Autodesk Inventor part; units mm, degrees
ref_plane "YZ Plane" through (0, 0, 0) normal (1, 0, 0) x (0, 1, 0)
ref_plane "XZ Plane" through (0, 0, 0) normal (0, 1, 0) x (-1, 0, 0)
ref_plane "XY Plane" through (0, 0, 0) normal (0, 0, 1) x (1, 0, 0)
sketch "Sketch1" plane through (0, 0, 0) normal (0, 0, 1) x (1, 0, 0)
  line L0 (0, 0) -> (175, 0)
  line L1 (0, 0) -> (0, 68)
  line L2 (0, 68) -> (-5, 68)
  line L3 (-5, 68) -> (-5, -5)
  line L4 (-5, -5) -> (180, -5)
  line L5 (180, -5) -> (180, 68)
  line L6 (180, 68) -> (175, 68)
  line L7 (175, 68) -> (175, 0)
  dimension "d0" = 175
  dimension "d1" = 68
  dimension "d2" = 5
  dimension "d3" = 73
  dimension "d4" = 185
  dimension "d5" = 73
  dimension "d6" = 5
extrude "Outline" add sketch "Sketch1" along normal blind 30
sketch "Sketch2" plane through (-5, -5, 0) normal (-1, 0, 0) x (0, 0, 1)
  line L0 (0, 73) -> (30, 73) construction
  line L1 (15, 73) -> (15, 43) construction
  line L2 (5, 22.5) -> (25, 22.5)
  line L3 (25, 22.5) -> (25, 63.5)
  line L4 (25, 63.5) -> (5, 63.5)
  line L5 (5, 63.5) -> (5, 22.5)
  line L6 (5, 22.5) -> (25, 63.5) construction
  line L7 (25, 22.5) -> (5, 63.5) construction
  line L8 (5, 63.5) -> (5, 67.5) construction
  line L9 (5, 67.5) -> (10, 67.5) construction
  line L10 (25, 63.5) -> (25, 67.5) construction
  line L11 (25, 67.5) -> (20, 67.5) construction
  line L12 (5, 22.5) -> (5, 18.5) construction
  line L13 (5, 18.5) -> (10, 18.5) construction
  line L14 (25, 22.5) -> (25, 18.5) construction
  line L15 (25, 18.5) -> (20, 18.5) construction
  circle A0 centre (10, 67.5) radius 2
  circle A1 centre (20, 67.5) radius 2
  circle A2 centre (10, 18.5) radius 2
  circle A3 centre (20, 18.5) radius 2
  point P0 (0, 5)
  dimension "d9" = 30
  dimension "d10" = 20
  dimension "d11" = 41
  dimension "d12" = 4
  dimension "d13" = 5
  dimension "d14" = 4
  dimension "d15" = 5
  dimension "d16" = 4
  dimension "d17" = 5
  dimension "d18" = 4
  dimension "d19" = 5
  dimension "d20" = 4
  dimension "d21" = 4
  dimension "d22" = 4
  dimension "d23" = 4
extrude "Servo Mount" cut sketch "Sketch2" against normal blind 10
sketch "Sketch3" plane through (175, 0, 0) normal (-1, 0, 0) x (0, 0, 1)
  line L0 (5, 58.5) -> (25, 58.5) construction
  line L1 (15, 58.5) -> (15, 47.5) construction
  circle A0 centre (15, 47.5) radius 10.75
  point P0 (0, 0)
  dimension "d26" = 11
  dimension "d27" = 21.5
extrude "Idler Mount" cut sketch "Sketch3" against normal blind 14.5
sketch "Sketch4" plane through (-5, -5, 0) normal (0, -1, 0) x (1, 0, 0)
  line L0 (0, 25) -> (0, 5) construction
  line L1 (99.5, 14.2941) -> (99.5, 15.7059)
  line L2 (60.5, 15.7059) -> (60.5, 14.2941)
  line L3 (79.2941, 34.5) -> (80.7059, 34.5)
  line L4 (80.7059, -4.5) -> (79.2941, -4.5)
  line L5 (84.5, 22.5) -> (84.5, 21.5)
  line L6 (84.5, 8.5) -> (84.5, 7.5)
  line L7 (75.5, 7.5) -> (75.5, 8.5)
  line L8 (75.5, 21.5) -> (75.5, 22.5)
  line L9 (72.5, 10.5) -> (73.5, 10.5)
  line L10 (86.5, 10.5) -> (87.5, 10.5)
  line L11 (87.5, 19.5) -> (86.5, 19.5)
  line L12 (73.5, 19.5) -> (72.5, 19.5)
  arc A0 (73.5, 19.5) -> (75.5, 21.5) centre (73.5, 21.5) ccw
  arc A1 (84.5, 21.5) -> (86.5, 19.5) centre (86.5, 21.5) ccw
  arc A2 (86.5, 10.5) -> (84.5, 8.5) centre (86.5, 8.5) ccw
  arc A3 (75.5, 8.5) -> (73.5, 10.5) centre (73.5, 8.5) ccw
  line L13 (84.5, 22.5) -> (82.6755, 32.8473)
  line L14 (75.5, 22.5) -> (77.3245, 32.8473)
  line L15 (87.5, 10.5) -> (97.8473, 12.3245)
  line L16 (87.5, 19.5) -> (97.8473, 17.6755)
  line L17 (72.5, 19.5) -> (62.1527, 17.6755)
  line L18 (72.5, 10.5) -> (62.1527, 12.3245)
  line L19 (75.5, 7.5) -> (77.3245, -2.8473)
  line L20 (84.5, 7.5) -> (82.6755, -2.8473)
  arc A4 (62.1527, 17.6755) -> (60.5, 15.7059) centre (62.5, 15.7059) ccw
  arc A5 (60.5, 14.2941) -> (62.1527, 12.3245) centre (62.5, 14.2941) ccw
  arc A6 (79.2941, 34.5) -> (77.3245, 32.8473) centre (79.2941, 32.5) ccw
  arc A7 (82.6755, 32.8473) -> (80.7059, 34.5) centre (80.7059, 32.5) ccw
  arc A8 (99.5, 15.7059) -> (97.8473, 17.6755) centre (97.5, 15.7059) ccw
  arc A9 (97.8473, 12.3245) -> (99.5, 14.2941) centre (97.5, 14.2941) ccw
  arc A10 (77.3245, -2.8473) -> (79.2941, -4.5) centre (79.2941, -2.5) ccw
  arc A11 (80.7059, -4.5) -> (82.6755, -2.8473) centre (80.7059, -2.5) ccw
  line L21 (80, 15) -> (66, 15) construction
  line L22 (80, 15) -> (80, 29) construction
  line L23 (80, 15) -> (94, 15) construction
  line L24 (80, 15) -> (80, 1) construction
  circle A12 centre (80, 29) radius 0.75
  circle A13 centre (66, 15) radius 0.75
  circle A14 centre (94, 15) radius 0.75
  circle A15 centre (80, 1) radius 0.75
  circle A16 centre (80, 15) radius 2.5
  point P0 (5, 0)
  dimension "d35" = 2
  dimension "d37" = 10
  dimension "d39" = 10
  dimension "d41" = 10
  dimension "d43" = 10
  dimension "d45" = 10
  dimension "d47" = 10
  dimension "d49" = 10
  dimension "d51" = 10
  dimension "d52" = 2
  dimension "d53" = 2
  dimension "d54" = 80
  dimension "d55" = 6.5
  dimension "d56" = 6.5
  dimension "d57" = 14
  dimension "d58" = 14
  dimension "d59" = 14
  dimension "d60" = 14
  dimension "d61" = 1.5
  dimension "d62" = 1.5
  dimension "d63" = 1.5
  dimension "d64" = 1.5
  dimension "d70" = 5
extrude "Bottom Servo indent" cut sketch "Sketch4" against normal blind 2 contours A9 L15 L10 A2 L6 L20 A11 L4 A10 L19 L7 A3 L9 L18 A5 L2 A4 L17 L12 A0 L8 L14 A6 L3 A7 L13 L5 A1 L11 L16 A8 L1 | A16
extrude "Bottom Servo Mounting Holse" cut sketch "Sketch4" against normal blind 22 contours A12 | A13 | A14 | A15 | A16
fillet "Strengthening Fillet" radius 4 4 edges at (0, 0, 15) (175, 0, 15) (-5, -5, 15) (180, -5, 15)
fillet "Rounded Idler Post" radius 15 2 edges at (177.5, 68, 0) (177.5, 68, 30)
equation "\"d3\" = d1 + d2"
equation "\"d4\" = d0 + 2 * d2"
equation "\"d5\" = d3"
equation "\"d6\" = d2"
equation "\"d14\" = d12"
equation "\"d15\" = d13"
equation "\"d16\" = d12"
equation "\"d17\" = d13"
equation "\"d18\" = d12"
equation "\"d19\" = d13"
equation "\"d39\" = d37"
equation "\"d41\" = d37"
equation "\"d43\" = d37"
equation "\"d45\" = d37"
equation "\"d47\" = d37"
equation "\"d49\" = d37"
equation "\"d51\" = d37"
equation "\"d58\" = d57"
equation "\"d59\" = d57"
equation "\"d60\" = d57"
equation "\"d62\" = d61"
equation "\"d63\" = d61"
equation "\"d64\" = d61"
properties part number "outerGantry" material "PET Plastic"
Input: part model. Units: mm. Frame: model coordinates. A direction names the side the tool comes from. Round coordinates to 2 decimals unless told otherwise and drop trailing zeros. Order: outer loops, then holes, each group sorted by start corner. A loop starts at its lowest first (then second) coordinate and runs counter-clockwise, first axis right, second up. Notation, with made-up numbers: (-30, 62.25) - (14, 62.25) arc R23 cw to (14, 87.25) - close; hole circle Ø3 at (-9, 0.25). An arc over 180 degrees is marked (long way). Answer in a Markdown table with one row per item.
Item 1: Pin query (flat end, axial travel): pin 1 (3 mm diameter, centred on x = 159.5, z = 4.5, fed in from +Y); pin 2 (1.6 mm diameter, centred on y = -4.5, z = 15, fed in from +X); pin 3 (6.5 mm diameter, centred on x = 75, z = 15, fed in from -Y). Return the tip coordinate at first contact, or that it passes through.
Model answer:
| item | result |
|---|---|
| pin 1 | stops at y = 0 |
| pin 2 | stops at x = 178.95 |
| pin 3 | stops at y = -3 |
Item 2: Section query C-C (y = 51). Return the cut outline in (x, z), then the cut area to 3 significant figures.
Model answer:
| item | result |
|---|---|
| outline | (-5, 0) - (0, 0) - (0, 5) - (-5, 5) - close; (-5, 25) - (0, 25) - (0, 30) - (-5, 30) - close; (175, 0) - (180, 0) - (180, 4.84) - (175, 4.84) - close; (175, 25.16) - (180, 25.16) - (180, 30) - (175, 30) - close |
| area | 98.4 mm² |
Item 3: Section query A-A (y = 34). Return the cut outline in (x, z).
Model answer:
| item | result |
|---|---|
| outline | (-5, 0) - (0, 0) - (0, 5) - (-5, 5) - close; (-5, 25) - (0, 25) - (0, 30) - (-5, 30) - close; (175, 0) - (180, 0) - (180, 30) - (175, 30) - close |
Item 4: Line query: line 1 (Z direction, x = 75, y = -0.65); line 2 (X direction, y = 48, z = 28.5); line 3 (Y direction, x = 80, z = 8.5). Output: solid intervals per line, ascending.
Model answer:
| item | result |
|---|---|
| line 1 | z = 0 to 0.25, 1.75 to 12.5, 17.5 to 28.25, 29.75 to 30 |
| line 2 | x = -5 to 0, 175 to 180 |
| line 3 | y = -5 to 0 |
Item 5: Section query B-B (y = 13.5). Return the cut outline in (x, z), then the cut area to 3 significant figures.
Model answer:
| item | result |
|---|---|
| outline | (-5, 0) - (0, 0) - (0, 8) - (-5, 8) - close; (-5, 12) - (0, 12) - (0, 18) - (-5, 18) - close; (-5, 22) - (0, 22) - (0, 30) - (-5, 30) - close; (175, 0) - (180, 0) - (180, 30) - (175, 30) - close |
| area | 260 mm² |
Item 6: Section query D-D (x = 32). Return the cut outline in (y, z).
Model answer:
| item | result |
|---|---|
| outline | (-5, 0) - (0, 0) - (0, 30) - (-5, 30) - close |
Item 7: Mould query, pull axis Y, two halves, no side actions, for faces 1 (the cylindrical face through (-2.535, 64.483, 19.74)), 2 (the flat face through (-5, 34, 4.8)), 3 (the cylindrical face through (177.46, 63.72, 4.51)), 4 (the cylindrical face through (-2.535, 14.852, 18.526)). Classes: released by +Y, released by -Y, zero draft, split by the parting line, or undercut.
Model answer:
| item | result |
|---|---|
| face 1 | undercut |
| face 2 | zero draft |
| face 3 | released by +Y |
| face 4 | undercut |
Item 8: Reachability of faces 5 (the cylindrical face through (177.46, 63.49, 25.72)), 6 (the flat face through (80, -1, 30)), 7 (the flat face through (76.4, -3, 17.3)), 8 (the cylindrical face through (1.141, 1.203, 15.21)), 9 (the cylindrical face through (-2.535, 15.483, 9.74)) from +Z, -Z, +X, -X, +Y, -Y: full face, straight path, thin tool, end or side. Return the list, or none.
Model answer:
| item | result |
|---|---|
| face 5 | +Z, +X, +Y |
| face 6 | +Z, +X, -X, +Y, -Y |
| face 7 | -Y |
| face 8 | +Z, -Z, +Y |
| face 9 | -X |
